from build123d import *

# Parameters (mm, degrees)
SKETCH_1_W               = 17
SKETCH_1_H               = 40
EXTRUDE_1_DEPTH          = 50
SKETCH_2_W               = 17
SKETCH_2_H               = 1
CUT_EXTRUDE_1_DEPTH      = 67.2495283
SKETCH_4_W               = 0.5
SKETCH_4_H               = 39
EXTRUDE_2_DEPTH          = 50
SKETCH_5_R               = 15.5
CUT_EXTRUDE_2_DEPTH      = 17.5
CUT_EXTRUDE_3_DEPTH      = 17.5
CUT_EXTRUDE_4_DEPTH      = 3
CUT_EXTRUDE_START        = -64
CUT_EXTRUDE_7_DEPTH      = 64
SKETCH_9_W               = 5
SKETCH_9_H               = 3
EXTRUDE_3_DEPTH          = 17.5
CUT_EXTRUDE_8_DEPTH      = 54.087192429
CUT_EXTRUDE_8_DEPTH_BACK = 54.087192429
CUT_EXTRUDE_10_REACH     = 51.07
CUT_EXTRUDE_11_REACH     = 55.087


with BuildPart() as part:
    # 草图1 → 凸台-拉伸1 (new body)
    with BuildSketch(Plane(origin=(0, 0, 0), x_dir=(1, 0, 0), z_dir=(0, 1, 0))):
        with Locations((8.5, -20)):
            Rectangle(SKETCH_1_W, SKETCH_1_H)
    extrude(amount=EXTRUDE_1_DEPTH)

    # 草图2 → 切除-拉伸1 (cut, through all)
    with BuildSketch(Plane.XZ):
        with Locations((8.5, 39.5)):
            Rectangle(SKETCH_2_W, SKETCH_2_H)
    extrude(amount=-CUT_EXTRUDE_1_DEPTH, mode=Mode.SUBTRACT)

    # 草图4 → 凸台-拉伸2 (add)
    with BuildSketch(Plane.XZ):
        with Locations((-0.25, 19.5)):
            Rectangle(SKETCH_4_W, SKETCH_4_H)
    extrude(amount=-EXTRUDE_2_DEPTH)

    # 草图5 → 切除-拉伸2 (cut)
    with BuildSketch(Plane(origin=(17, 0, 0), x_dir=(0, 0, -1), z_dir=(1, 0, 0))):
        with Locations((-22, 4.5)):
            Circle(SKETCH_5_R)
    extrude(amount=-CUT_EXTRUDE_2_DEPTH, mode=Mode.SUBTRACT)

    # 草图6 → 切除-拉伸3 (cut)
    with BuildSketch(Plane(origin=(17, 0, 0), x_dir=(0, 0, -1), z_dir=(1, 0, 0))):
        Polygon((0, 3), (0, 24), (0, 50), (-39, 50), (-39, 24), (-22, 24), (-5, 24), (-5, 3), align=None)
    extrude(amount=-CUT_EXTRUDE_3_DEPTH, mode=Mode.SUBTRACT)

    # 草图7 → 切除-拉伸4 (cut)
    with BuildSketch(Plane(origin=(0, 3, 0), x_dir=(1, 0, 0), z_dir=(0, 1, 0))):
        with BuildLine():
            ThreePointArc((8.25, -0.9), (6.65, -2.5), (8.25, -4.1))
            Line((8.25, -4.1), (8.25, -0.9))
        make_face()
        with BuildLine():
            Line((8.25, -0.9), (8.25, -4.1))
            ThreePointArc((8.25, -4.1), (9.38137085, -3.63137085), (9.85, -2.5))
            ThreePointArc((9.85, -2.5), (9.38137085, -1.36862915), (8.25, -0.9))
        make_face()
    extrude(amount=-CUT_EXTRUDE_4_DEPTH, mode=Mode.SUBTRACT)

    # 草图8 → 切除-拉伸7 (cut)
    with BuildSketch(Plane.ZY.offset(0.5).offset(CUT_EXTRUDE_START)):
        with BuildLine():
            Line((5, 3), (5, 4.5))
            Line((5, 4.5), (-8.613521725, 4.5))
            Line((-8.613521725, 4.5), (17.256515703, -28.446816898))
            Line((17.256515703, -28.446816898), (39, 0))
            Line((39, 0), (36.832396974, 0))
            ThreePointArc((36.832396974, 0), (22, -11), (7.167603026, 0))
            Line((7.167603026, 0), (0, 0))
            Line((0, 0), (0, 3))
            Line((0, 3), (5, 3))
        make_face()
        with BuildLine():
            ThreePointArc((7.167603026, 0), (6.667809141, 2.225373998), (6.5, 4.5))
            Line((6.5, 4.5), (5, 4.5))
            Line((5, 4.5), (5, 3))
            Line((5, 3), (0, 3))
            Line((0, 3), (0, 0))
            Line((0, 0), (7.167603026, 0))
        make_face()
        with BuildLine():
            Line((37.5, 4.5), (22, 4.5))
            Line((22, 4.5), (6.5, 4.5))
            ThreePointArc((6.5, 4.5), (6.667809141, 2.225373998), (7.167603026, 0))
            ThreePointArc((7.167603026, 0), (22, -11), (36.832396974, 0))
            ThreePointArc((36.832396974, 0), (37.332190859, 2.225373998), (37.5, 4.5))
        make_face()
        with BuildLine():
            Line((6.5, 4.5), (22, 4.5))
            Line((22, 4.5), (37.5, 4.5))
            ThreePointArc((37.5, 4.5), (22, 20), (6.5, 4.5))
        make_face()
        with BuildLine():
            Line((39, 4.5), (37.5, 4.5))
            ThreePointArc((37.5, 4.5), (37.332190859, 2.225373998), (36.832396974, 0))
            Line((36.832396974, 0), (39, 0))
            Line((39, 0), (39, 4.5))
        make_face()
    extrude(amount=CUT_EXTRUDE_7_DEPTH, mode=Mode.SUBTRACT)

    # 草图9 → 凸台-拉伸3 (add)
    with BuildSketch(Plane.ZY.offset(0.5)):
        with Locations((41.5, 8.978432147)):
            Rectangle(SKETCH_9_W, SKETCH_9_H)
        with Locations((2.5, 8.978432147)):
            Rectangle(SKETCH_9_W, SKETCH_9_H)
    extrude(amount=-EXTRUDE_3_DEPTH)

    # 草图10 → 切除-拉伸8 (cut, two sides: drawn at the far end of the back side and taken through both)
    with BuildSketch(Plane.ZY.offset(0.5).offset(-CUT_EXTRUDE_8_DEPTH_BACK)):
        with BuildLine():
            Line((5, 24), (5, 14.052486587))
            ThreePointArc((5, 14.052486587), (12.151738439, 21.330381583), (22, 24))
            Line((22, 24), (5, 24))
        make_face()
        with BuildLine():
            Line((39, 24), (22, 24))
            ThreePointArc((22, 24), (31.848261561, 21.330381583), (39, 14.052486587))
            Line((39, 14.052486587), (39, 24))
        make_face()
    extrude(amount=CUT_EXTRUDE_8_DEPTH + CUT_EXTRUDE_8_DEPTH_BACK, mode=Mode.SUBTRACT)

    # 草图12 → 切除-拉伸10 (cut, up to next)
    with BuildSketch(Plane(origin=(0, 10.478432147, 0), x_dir=(1, 0, 0), z_dir=(0, 1, 0)), mode=Mode.PRIVATE) as cut_extrude_10_sk1:
        with BuildLine():
            ThreePointArc((9.85, -41.5), (9.38137085, -40.36862915), (8.25, -39.9))
            Line((8.25, -39.9), (8.25, -43.1))
            ThreePointArc((8.25, -43.1), (9.38137085, -42.63137085), (9.85, -41.5))
        make_face()
    cut_extrude_10_tool1 = extrude(cut_extrude_10_sk1.sketch, amount=-CUT_EXTRUDE_10_REACH, mode=Mode.PRIVATE) & part.part
    # 草图12 → 切除-拉伸10 (cut, up to next)
    with BuildSketch(Plane(origin=(0, 10.478432147, 0), x_dir=(1, 0, 0), z_dir=(0, 1, 0)), mode=Mode.PRIVATE) as cut_extrude_10_sk2:
        with BuildLine():
            Line((8.25, -43.1), (8.25, -39.9))
            ThreePointArc((8.25, -39.9), (6.65, -41.5), (8.25, -43.1))
        make_face()
    cut_extrude_10_tool2 = extrude(cut_extrude_10_sk2.sketch, amount=-CUT_EXTRUDE_10_REACH, mode=Mode.PRIVATE) & part.part
    # 草图12 → 切除-拉伸10 (cut, up to next)
    with BuildSketch(Plane(origin=(0, 10.478432147, 0), x_dir=(1, 0, 0), z_dir=(0, 1, 0)), mode=Mode.PRIVATE) as cut_extrude_10_sk3:
        with BuildLine():
            ThreePointArc((9.85, -41.5), (9.38137085, -40.36862915), (8.25, -39.9))
            Line((8.25, -39.9), (8.25, -43.1))
            ThreePointArc((8.25, -43.1), (9.38137085, -42.63137085), (9.85, -41.5))
        make_face()
    cut_extrude_10_tool3 = extrude(cut_extrude_10_sk3.sketch, amount=-CUT_EXTRUDE_10_REACH, mode=Mode.PRIVATE) & part.part
    # 草图12 → 切除-拉伸10 (cut, up to next)
    with BuildSketch(Plane(origin=(0, 10.478432147, 0), x_dir=(1, 0, 0), z_dir=(0, 1, 0)), mode=Mode.PRIVATE) as cut_extrude_10_sk4:
        with BuildLine():
            Line((8.25, -43.1), (8.25, -39.9))
            ThreePointArc((8.25, -39.9), (6.65, -41.5), (8.25, -43.1))
        make_face()
    cut_extrude_10_tool4 = extrude(cut_extrude_10_sk4.sketch, amount=-CUT_EXTRUDE_10_REACH, mode=Mode.PRIVATE) & part.part
    # 草图12 → 切除-拉伸10 (cut, up to next)
    with BuildSketch(Plane(origin=(0, 10.478432147, 0), x_dir=(1, 0, 0), z_dir=(0, 1, 0)), mode=Mode.PRIVATE) as cut_extrude_10_sk5:
        with BuildLine():
            ThreePointArc((9.85, -2.5), (9.38137085, -1.36862915), (8.25, -0.9))
            Line((8.25, -0.9), (8.25, -4.1))
            ThreePointArc((8.25, -4.1), (9.38137085, -3.63137085), (9.85, -2.5))
        make_face()
    cut_extrude_10_tool5 = extrude(cut_extrude_10_sk5.sketch, amount=-CUT_EXTRUDE_10_REACH, mode=Mode.PRIVATE) & part.part
    # 草图12 → 切除-拉伸10 (cut, up to next)
    with BuildSketch(Plane(origin=(0, 10.478432147, 0), x_dir=(1, 0, 0), z_dir=(0, 1, 0)), mode=Mode.PRIVATE) as cut_extrude_10_sk6:
        with BuildLine():
            Line((8.25, -4.1), (8.25, -0.9))
            ThreePointArc((8.25, -0.9), (6.65, -2.5), (8.25, -4.1))
        make_face()
    cut_extrude_10_tool6 = extrude(cut_extrude_10_sk6.sketch, amount=-CUT_EXTRUDE_10_REACH, mode=Mode.PRIVATE) & part.part
    # 草图12 → 切除-拉伸10 (cut, up to next)
    with BuildSketch(Plane(origin=(0, 10.478432147, 0), x_dir=(1, 0, 0), z_dir=(0, 1, 0)), mode=Mode.PRIVATE) as cut_extrude_10_sk7:
        with BuildLine():
            ThreePointArc((9.85, -2.5), (9.38137085, -1.36862915), (8.25, -0.9))
            Line((8.25, -0.9), (8.25, -4.1))
            ThreePointArc((8.25, -4.1), (9.38137085, -3.63137085), (9.85, -2.5))
        make_face()
    cut_extrude_10_tool7 = extrude(cut_extrude_10_sk7.sketch, amount=-CUT_EXTRUDE_10_REACH, mode=Mode.PRIVATE) & part.part
    # 草图12 → 切除-拉伸10 (cut, up to next)
    with BuildSketch(Plane(origin=(0, 10.478432147, 0), x_dir=(1, 0, 0), z_dir=(0, 1, 0)), mode=Mode.PRIVATE) as cut_extrude_10_sk8:
        with BuildLine():
            Line((8.25, -4.1), (8.25, -0.9))
            ThreePointArc((8.25, -0.9), (6.65, -2.5), (8.25, -4.1))
        make_face()
    cut_extrude_10_tool8 = extrude(cut_extrude_10_sk8.sketch, amount=-CUT_EXTRUDE_10_REACH, mode=Mode.PRIVATE) & part.part
    add(cut_extrude_10_tool1.solids().sort_by_distance((8.929061, 10.478432, 41.5))[0], mode=Mode.SUBTRACT)
    add(cut_extrude_10_tool2.solids().sort_by_distance((7.570939, 10.478432, 41.5))[0], mode=Mode.SUBTRACT)
    add(cut_extrude_10_tool3.solids().sort_by_distance((8.929061, 10.478432, 41.5))[0], mode=Mode.SUBTRACT)
    add(cut_extrude_10_tool4.solids().sort_by_distance((7.570939, 10.478432, 41.5))[0], mode=Mode.SUBTRACT)
    add(cut_extrude_10_tool5.solids().sort_by_distance((8.929061, 10.478432, 2.5))[0], mode=Mode.SUBTRACT)
    add(cut_extrude_10_tool6.solids().sort_by_distance((7.570939, 10.478432, 2.5))[0], mode=Mode.SUBTRACT)
    add(cut_extrude_10_tool7.solids().sort_by_distance((8.929061, 10.478432, 2.5))[0], mode=Mode.SUBTRACT)
    add(cut_extrude_10_tool8.solids().sort_by_distance((7.570939, 10.478432, 2.5))[0], mode=Mode.SUBTRACT)

    # 草图13 → 切除-拉伸11 (cut, up to next)
    with BuildSketch(Plane(origin=(17, 0, 0), x_dir=(0, 0, -1), z_dir=(1, 0, 0)), mode=Mode.PRIVATE) as cut_extrude_11_sk1:
        Polygon((-39, 7.478432147), (-37.21114532, 7.478432147), (-37.5, 4.5), (-39, 4.5), align=None)
    cut_extrude_11_tool1 = extrude(cut_extrude_11_sk1.sketch, amount=-CUT_EXTRUDE_11_REACH, mode=Mode.PRIVATE) & part.part
    # 草图13 → 切除-拉伸11 (cut, up to next)
    with BuildSketch(Plane(origin=(17, 0, 0), x_dir=(0, 0, -1), z_dir=(1, 0, 0)), mode=Mode.PRIVATE) as cut_extrude_11_sk2:
        Polygon((-5, 7.478432147), (-6.78885468, 7.478432147), (-6.5, 4.5), (-5, 4.5), align=None)
    cut_extrude_11_tool2 = extrude(cut_extrude_11_sk2.sketch, amount=-CUT_EXTRUDE_11_REACH, mode=Mode.PRIVATE) & part.part
    add(cut_extrude_11_tool1.solids().sort_by_distance((17, 6.032815, 38.175672))[0], mode=Mode.SUBTRACT)
    add(cut_extrude_11_tool2.solids().sort_by_distance((17, 6.032815, 5.824328))[0], mode=Mode.SUBTRACT)


solid = part.part
Model file for the job. Use its own axes, mm. A direction names the side the tool comes from. Coordinates: 2 decimals unless noted, no trailing zeros. Loops run counter-clockwise (first coordinate to the right, second up) from the corner with the lowest first, then second, coordinate; pieces in that order, holes last. Notation, with made-up numbers: (30.25, 29) -> (84.25, 29) arc R22 ccw to (84.25, 58) -> close; hole circle Ø1 at (-24.75, 71). An arc over 180 degrees is marked (long way). Use one line per item in the form item = value. Start each with the question number.
(1) Cut at C-C on y = 12.5. Give the cut face in (x, z).
(2) Cut at D-D on y = 17.25. Give the cut face in (x, z).
(3) Cut at B-B on x = 5.25. Give the cut face in (y, z).
(4) Pull direction Z, two halves, no side cores. Call faces 1 (the flat face through (8, 9, 0)), 2 (the flat face through (8, 12, 39)), 3 (the flat face through (-0.5, 21, 22)), 4 (the cylindrical face through (8, 20, 22)): pulls with the +Z half, pulls with the -Z half, needs draft (parallel to the pull), parting line crosses it, or undercut.
(5) Cut at A-A on y = 8.5. Give the cut face in (x, z).
(6) Tool access for faces 5 (the flat face through (17, 21, 22)), 6 (the flat face through (8, 12, 5)), 7 (the flat face through (10, 10.478, 41)): list every direction of +Z, -Z, +X, -X, +Y, -Y with a clear straight run to the whole face (end or side of a thin tool).
(7) Probe probe 1 along Z at (x, y) = (9.25, 8); probe 2 along Z at (x, y) = (6.5, 16.75); probe 3 along Y at (x, z) = (2.25, 40). List the from-to ranges inside material, lowest first. Write a range as from..to.
(8) Flat gauge pins, fed straight in: pin 1 (5 mm diameter, centred on x = 13, z = 17, fed in from -Y); pin 2 (2.5 mm diameter, centred on x = 5, z = 3, fed in from +Y); pin 3 (10 mm diameter, centred on x = 11, z = 6, fed in from +Y); pin 4 (5 mm diameter, centred on y = 16.5, z = 6, fed in from -X). Where does each tip first touch, or does it go through?
Values:
q1.outline = (-0.5, 5) -> (17, 5) -> (17, 8.72) -> (-0.5, 8.72) -> close; (-0.5, 35.28) -> (17, 35.28) -> (17, 39) -> (-0.5, 39) -> close
q2.outline = (-0.5, 7.25) -> (17, 7.25) -> (17, 13.19) -> (-0.5, 13.19) -> close; (-0.5, 30.81) -> (17, 30.81) -> (17, 36.75) -> (-0.5, 36.75) -> close
q3.outline = (7.48, 0) -> (10.48, 0) -> (10.48, 5) -> (14.05, 5) arc R19.5 ccw to (14.05, 39) -> (10.48, 39) -> (10.48, 44) -> (7.48, 44) -> (7.48, 37.21) arc R15.5 cw to (7.48, 6.79) -> close
q4.face_1 = pulls with the -Z half
q4.face_2 = pulls with the +Z half
q4.face_3 = needs draft
q4.face_4 = undercut
q5.outline = (-0.5, 0) -> (17, 0) -> (17, 7.03) -> (-0.5, 7.03) -> close; (-0.5, 36.97) -> (17, 36.97) -> (17, 44) -> (-0.5, 44) -> close; hole circle Ø3.2 at (8.25, 2.5); hole circle Ø3.2 at (8.25, 41.5)
q6.face_5 = +Z, -Z, +X, +Y, -Y
q6.face_6 = -Z, +X, -X, +Y
q6.face_7 = +Z, +X, -X, +Y
q7.probe_1 = 0..1.25, 3.75..6.9, 37.1..40.25, 42.75..44
q7.probe_2 = 6.83..12.5, 31.5..37.17
q7.probe_3 = 7.48..10.48
q8.pin_1 = 18.06
q8.pin_2 = 10.48
q8.pin_3 = 20.6
q8.pin_4 = -0.5
